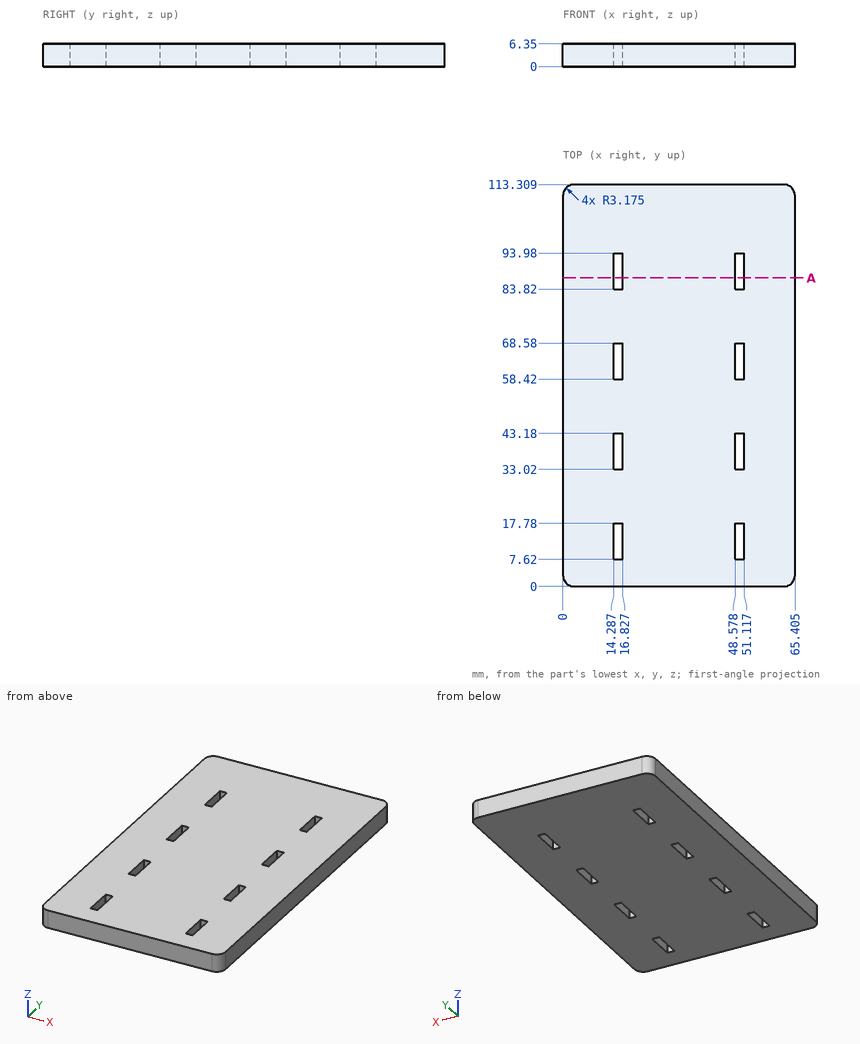
Geometry: see drawing. Coordinates: mm, zero at the bounding-box minimum. Give positions to 0.01 mm unless a question says otherwise; leave off trailing zeros. Write item = value, one per line.
Q1. Material intervals for line 1 (X direction, y = 41.5, z = 4) (1 decimal); line 2 (Y direction, x = 49, z = 5.5), sorted ascending. Write a range as from..to.
Data:
line_1 = 0..14.3, 16.8..48.6, 51.1..65.4
line_2 = 0..7.62, 17.78..33.02, 43.18..58.42, 68.58..83.82, 93.98..113.31
Q2. Cut plane A-A, the plane y = 87. State how many separate pieces and enclosed holes the cut face has, and give its area (3 significant figures).
Data:
separate_pieces = 3
enclosed_holes = 0
area = 383 mm^2
Q3. Pin query (flat end, axial travel): pin 1 (12 mm diameter, centred on x = 53.5, y = 49, fed in from -Z). Return the tip coordinate at first contact, or that it passes through.
Data:
pin_1 = 0
